CAD build for the part. Positions are in the model's coordinates, mm. A direction names the side the tool comes from. Round coordinates to 2 decimals unless told otherwise and drop trailing zeros. Write each loop counter-clockwise with the first axis right and the second up, starting at its lowest first coordinate (ties: lowest second). Pieces come first, ordered by that corner, then holes. Notation, with made-up numbers: (88.25, -8) - (137.25, -8) arc R29 cw to (137.25, 28) - close; hole circle Ø9 at (-36, 37.5). An arc over 180 degrees is marked (long way). Put each result on its own line as item: value. Start each with the question number.
Item 1: Cut at B-B (z = 18). Give the cut face in (x, y).
Item 2: Mould opens along Y. For faces 4 (the flat face through (35.76, 6.88, 12.52)), 5 (the flat face through (2, -9, 0)), 6 (the flat face through (4.03, 39.25, 12.52)) say: released by +Y, released by -Y, zero draft, split by the parting line, or undercut.
Item 3: Pin check, flat tips, straight feed: pin 1 Ø6 at (x, z) = (34, 20) entering from +Y; pin 2 Ø12 at (y, z) = (-28, 16.5) entering from -X; pin 3 Ø6 at (y, z) = (4.5, 9) entering from +X; pin 4 Ø8 at (x, y) = (22, -32) entering from -Z. Stop position of each tip, or through.
Item 4: 3-axis set-ups, long thin cutter, end or side, ignore diameter. For faces 1 (the flat face through (-24, 29.317, 13)), 2 (the flat face through (-24, -44.891, 13)), 3 (the flat face through (-32.729, 9.754, 12.522)): which of +Z, -Z, +X, -X, +Y, -Y reach the whole face in a straight line?
Item 5: Cut at D-D (y = -27). Give the cut face in (x, z).
Item 6: Cut at C-C (x = -12). Give the cut face in (y, z), and give its area (3 significant figures).
Item 7: Cut at A-A (x = 32). Give the cut face in (y, z), and give its area (3 significant figures).
Item 8: Drill centre lines: line 1 (Y direction, x = -26, z = 3.5); line 2 (Y direction, x = 20, z = 1.5); line 3 (Y direction, x = -33, z = 23.5). Where is each one in solid material? Low to high. Write a range as from..to.
```python
from build123d import *

# Parameters (mm, degrees)
F1_DEPTH = 25.4


with BuildPart() as f1:
    # F0 (on Top) → F1 (new body)
    with BuildSketch(Plane.XY):
        Polygon((-8.186579082, 29.3166413903), (-40.9211441875, 29.3166413903), (-24.3044075905, -10.3651176924), align=None)
        Polygon((0, 49.4718290865), (-8.186579082, 29.3166413903), (7.9457961573, 29.3166413903), align=None)
        Polygon((7.9457961573, 29.3166413903), (-8.186579082, 29.3166413903), (-24.3044075905, -10.3651176924), (-9.8466492379, -44.8911078274), (11.169333611, -44.8911078274), (25.3944805374, -14.9434304482), align=None)
        Polygon((-9.8466492379, -44.8911078274), (-24.3044075905, -10.3651176924), (-38.3280799513, -44.8911078274), align=None)
        Polygon((46.4180149138, 29.3166413903), (7.9457961573, 29.3166413903), (25.3944805374, -14.9434304482), align=None)
        Polygon((11.169333611, -44.8911078274), (-9.8466492379, -44.8911078274), (0, -68.4054940939), align=None)
        Polygon((37.2007779247, -44.8911078274), (25.3944805374, -14.9434304482), (11.169333611, -44.8911078274), align=None)
    extrude(amount=F1_DEPTH)


solid = f1.part
```
Output values:
1. outline: (-40.92, 29.32) - (-24.3, -10.37) - (-38.33, -44.89) - (-9.85, -44.89) - (0, -68.41) - (11.17, -44.89) - (37.2, -44.89) - (25.39, -14.94) - (46.42, 29.32) - (7.95, 29.32) - (0, 49.47) - (-8.19, 29.32) - close
2. face 4: undercut
2. face 5: zero draft
2. face 6: released by +Y
3. pin 1: y = 29.32
3. pin 2: x = -33.9
3. pin 3: x = 36.06
3. pin 4: z = 0
4. face 1: +Z, -Z, -X, +Y
4. face 2: +Z, -Z, -X, -Y
4. face 3: +Z, -Z, -X
5. outline: (-31.06, 0) - (30.15, 0) - (30.15, 25.4) - (-31.06, 25.4) - close
6. outline: (-44.89, 0) - (29.32, 0) - (29.32, 25.4) - (-44.89, 25.4) - close
6. area: 1,880 mm2
7. outline: (-44.89, 0) - (-31.7, 0) - (-31.7, 25.4) - (-44.89, 25.4) - close; (-1.04, 0) - (29.32, 0) - (29.32, 25.4) - (-1.04, 25.4) - close
7. area: 1,110 mm2
8. line 1: -44.89..-14.54, -6.32..29.32
8. line 2: -44.89..29.32
8. line 3: -44.89..-31.77, 10.4..29.32
